from build123d import *

# Parameters (mm, degrees)
SKETCH_1_W      = 150
SKETCH_1_H      = 150
EXTRUDE_1_DEPTH = 200
SHELL_1_T       = -20


with BuildPart() as part:
    # 草图1 → 凸台-拉伸1 (new body)
    with BuildSketch(Plane(origin=(0, 0, 0), x_dir=(1, 0, 0), z_dir=(0, 1, 0))):
        Rectangle(SKETCH_1_W, SKETCH_1_H)
    extrude(amount=EXTRUDE_1_DEPTH)

    # 抽壳1
    shell_1_openings = [part.faces().sort_by_distance(p)[0] for p in [
        (0, 100, 75),
    ]]
    offset(amount=SHELL_1_T, openings=shell_1_openings, kind=Kind.INTERSECTION)


solid = part.part
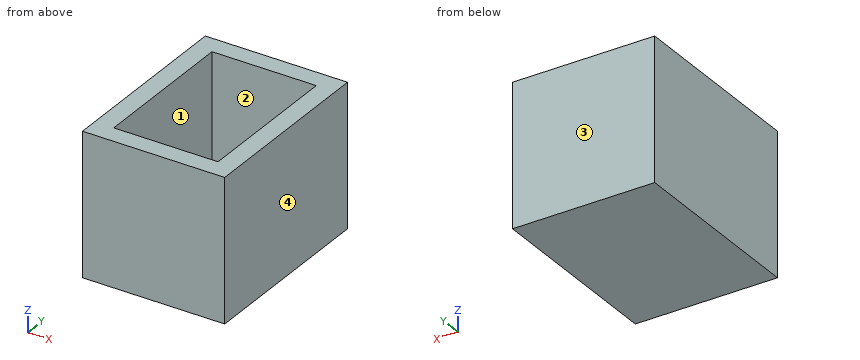
Model file for the job. Use its own axes, mm. Face numbers are marked on the shaded views. Give positions to 0.01 mm unless a question says otherwise; leave off trailing zeros. Write each loop counter-clockwise with the first axis right and the second up, starting at its lowest first coordinate (ties: lowest second). Pieces come first, ordered by that corner, then holes. Notation, with made-up numbers: M 9.5,35.25 L 25.5,35.25 A9 ccw 25.5,45.25 Z; hole C 6.25,60.25 d6. An arc over 180 degrees is marked long. One line per item, written item: value. Start each with the question number.
Q1. Drop flat-ended pins along their axis: pin 1 Ø12 at (x, z) = (-5, -42.5) entering from -Y; pin 2 Ø1.5 at (x, y) = (36.5, 74) entering from +Z. Give the stop position or say it passes through.
Q2. Saw through at B-B, the plane y = 59.5. Write the cut outline in (x, z), plus the area to 3 significant figures.
Q3. Saw through at A-A, the plane z = 59. Write the cut outline in (x, y), plus the area to 3 significant figures.
Q4. Two-plate mould, pull along Y, no slides. Class the marked faces 1, 2, 3 and 4: +Y half, -Y half, draft (parallel to the pull), parting line (faces both ways), or undercut.
Q5. Probe probe 1 along X at (y, z) = (59, 49.5); probe 2 along Y at (x, z) = (-52.5, -23); probe 3 along Z at (x, y) = (40.5, 34.5). List the from-to ranges inside material, lowest first. Write a range as [from, to].
Q6. Saw through at C-C, the plane x = -40. Write the cut outline in (y, z), plus the area to 3 significant figures.
Output values:
1. pin 1: stops at y = 0
1. pin 2: stops at z = -55
2. outline: M -75,-75 L 75,-75 L 75,75 L 55,75 L 55,-55 L -55,-55 L -55,75 L -75,75 Z
2. area: 8,200 mm²
3. outline: M -75,0 L 75,0 L 75,200 L -75,200 Z; hole M -55,20 L 55,20 L 55,180 L -55,180 Z
3. area: 12,400 mm²
4. face 1: undercut
4. face 2: undercut
4. face 3: +Y half
4. face 4: draft
5. probe 1: x = [-75, -55], [55, 75]
5. probe 2: y = [0, 20], [180, 200]
5. probe 3: z = [-75, -55]
6. outline: M 0,-75 L 200,-75 L 200,75 L 180,75 L 180,-55 L 20,-55 L 20,75 L 0,75 Z
6. area: 9,200 mm²
